Autodesk Inventor part; units mm, degrees
ref_plane "YZ Plane" through (0, 0, 0) normal (1, 0, 0) x (0, 1, 0)
ref_plane "XZ Plane" through (0, 0, 0) normal (0, 1, 0) x (-1, 0, 0)
ref_plane "XY Plane" through (0, 0, 0) normal (0, 0, 1) x (1, 0, 0)
sketch "Sketch1" plane through (0, 0, 0) normal (0, 1, 0) x (-1, 0, 0)
  line L0 (0, -37.5) -> (0, 0)
  line L1 (0, 0) -> (-74.5, 0)
  line L2 (-74.5, 0) -> (-74.5, -18)
  line L3 (-74.5, -18) -> (-15, -37.5)
  line L4 (-15, -37.5) -> (0, -37.5)
  dimension "d0" = 37.5
  dimension "d1" = 74.5
  dimension "d2" = 18
  dimension "d3" = 15
extrude "Extrusion1" add sketch "Sketch1" along normal blind 6.5
sketch "Sketch2" plane through (0, 0, 0) normal (0, -1, 0) x (1, 0, 0)
  line L0 (0, 0) -> (0, -37.5)
  line L1 (0, -37.5) -> (15, -37.5)
  line L2 (16.3, -23.5) -> (16.3, -28)
  line L3 (0, -28) -> (0, -23.5)
  line L4 (5, -21) -> (12.3, -21)
  line L5 (12.3, -30.5) -> (5, -30.5)
  line L6 (0, -23.5) -> (5, -23.5)
  line L7 (12.3, -23.5) -> (16.3, -23.5)
  line L8 (16.3, -28) -> (12.3, -28)
  line L9 (5, -28) -> (0, -28)
  line L10 (5, -30.5) -> (5, -28)
  line L11 (5, -23.5) -> (5, -21)
  line L12 (12.3, -21) -> (12.3, -23.5)
  line L13 (12.3, -28) -> (12.3, -30.5)
  point P0 (16.3, -25.75)
  dimension "d6" = 4.5
  dimension "d7" = 2.5
  dimension "d8" = 5
  dimension "d9" = 7.3
  dimension "d10" = 4
  dimension "d12" = 14
extrude "Extrusion2" cut sketch "Sketch2" against normal through all
sketch "Sketch3" plane through (0, 0, 0) normal (0, -1, 0) x (1, 0, 0)
  line L0 (74.5, -18) -> (74.5, 0)
  line L1 (74.5, 0) -> (0, 0)
  line L2 (66.5, 0) -> (58.5, 0)
  line L3 (58.5, 0) -> (58.5, 4.5)
  line L4 (60.5, 6.5) -> (64.5, 6.5)
  line L5 (66.5, 4.5) -> (66.5, 0)
  arc A0 (60.5, 6.5) -> (58.5, 4.5) centre (60.5, 4.5) ccw
  arc A1 (66.5, 4.5) -> (64.5, 6.5) centre (64.5, 4.5) ccw
  dimension "d15" = 2
  dimension "d16" = 8
  dimension "d17" = 6.5
  dimension "d18" = 8
extrude "Extrusion3" add sketch "Sketch3" against normal blind 6.5
sketch "Sketch4" plane through (0, 0, 0) normal (0, -1, 0) x (1, 0, 0)
  line L0 (58.5, 4.5) -> (58.5, 0)
  line L1 (58.5, 0) -> (0, 0)
  line L2 (48.75, 0) -> (53.25, 0)
  line L3 (53.25, -16.3) -> (48.75, -16.3)
  line L4 (55.75, -5) -> (55.75, -12.3)
  line L5 (46.25, -12.3) -> (46.25, -5)
  line L6 (46.25, -5) -> (48.75, -5)
  line L7 (53.25, -5) -> (55.75, -5)
  line L8 (55.75, -12.3) -> (53.25, -12.3)
  line L9 (48.75, -12.3) -> (46.25, -12.3)
  line L10 (48.75, -16.3) -> (48.75, -12.3)
  line L11 (48.75, -5) -> (48.75, 0)
  line L12 (53.25, 0) -> (53.25, -5)
  line L13 (53.25, -12.3) -> (53.25, -16.3)
  point P0 (51, -16.3)
  dimension "d21" = 4.5
  dimension "d22" = 2.5
  dimension "d23" = 5
  dimension "d24" = 4
  dimension "d25" = 7.3
  dimension "d26" = 7.5
extrude "Extrusion4" cut sketch "Sketch4" against normal through all
sketch "Sketch5" plane through (0, 0, 0) normal (0, -1, 0) x (1, 0, 0)
  line L0 (15, -37.5) -> (74.5, -18)
  line L1 (74.5, -18) -> (74.5, 0)
  line L2 (74.5, 0) -> (66.5, 0)
  arc A0 (71.9111, -18.8485) -> (57.845, -23.4584) centre (64.5, -20) ccw
  dimension "d29" = 15
  dimension "d30" = 20
  dimension "d31" = 10
extrude "Extrusion5" cut sketch "Sketch5" against normal through all
properties part number "x_carryage_brace_bottom"
CAD build for the part. Positions are in the model's coordinates, mm. A direction names the side the tool comes from. Give positions to 0.01 mm unless a question says otherwise; leave off trailing zeros. Loops run counter-clockwise (first coordinate to the right, second up) from the corner with the lowest first, then second, coordinate; pieces in that order, holes last. Notation, with made-up numbers: M 14,20 L 64,20 A17 ccw 64,49 Z; hole C -3,84.5 d8. An arc over 180 degrees is marked long. One line per question, with ' | ' between items. Start each with the question number.
1. Two-plate mould, pull along X, no slides. Class faces 1 (the face through (29, 6.5, -15)), 2 (the face through (48.75, 3, -3)), 3 (the face through (5, 3, -29)), 4 (the face through (0, 3, -12)): pulls with the +X half, pulls with the -X half, needs draft (parallel to the pull), parting line crosses it, or undercut.
2. 3-axis set-ups, long thin cutter, end or side, ignore diameter. For faces 5 (the face through (5, 3, -22)), 6 (the face through (2, 3, -23.5)), 7 (the face through (56, 3, 0)): which of +Z, -Z, +X, -X, +Y, -Y reach the whole face in a straight line?
3. Saw through at C-C on z = -13.5. Give the cut face in (x, y), plus the area to 3 significant figures.
4. Saw through at D-D on x = 38. Give the cut face in (y, z).
5. Probe L1, parallel to Z at x = 4, y = 1.25; L2, parallel to Z at x = 8.5, y = 4.75; L3, parallel to X at y = 2.5, z = -11. List the from-to ranges inside material, lowest first. Write a range as from..to.
6. Flat gauge pins, fed straight in: pin 1 (3 mm diameter, centred on x = 13.5, y = 4.5, fed in from +Z); pin 2 (2 mm diameter, centred on x = 48, y = 4.5, fed in from -Z); pin 3 (3.5 mm diameter, centred on y = 3, z = 2.5, fed in from +X); pin 4 (1 mm diameter, centred on x = 17, z = 1.5, fed in from +Y). Where does each tip first touch, or does it go through?
7. Saw through at B-B on x = 9. Give the cut face in (y, z), plus the area to 3 significant figures.
8. Saw through at A-A on z = -7. Give the cut face in (x, y).
Result sheet:
1) face 1: needs draft | face 2: undercut | face 3: undercut | face 4: pulls with the -X half
2) face 5: +Y, -Y | face 6: -X, +Y, -Y | face 7: +Z, -X, +Y, -Y
3) outline: M 0,0 L 48.75,0 L 48.75,6.5 L 0,6.5 Z; M 53.25,0 L 60.76,0 L 60.76,6.5 L 53.25,6.5 Z; M 68.24,0 L 74.5,0 L 74.5,6.5 L 68.24,6.5 Z | area: 406 mm^2
4) outline: M 0,-29.96 L 6.5,-29.96 L 6.5,0 L 0,0 Z
5) L1: z = -37.5..-28, -23.5..0 | L2: z = -37.5..-30.5, -21..0 | L3: x = 0..46.25, 55.75..74.5
6) pin 1: stops at z = 0 | pin 2: stops at z = -27.01 | pin 3: stops at x = 66.5 | pin 4: passes through
7) outline: M 0,-37.5 L 6.5,-37.5 L 6.5,-30.5 L 0,-30.5 Z; M 0,-21 L 6.5,-21 L 6.5,0 L 0,0 Z | area: 182 mm^2
8) outline: M 0,0 L 46.25,0 L 46.25,6.5 L 0,6.5 Z; M 55.75,0 L 74.5,0 L 74.5,6.5 L 55.75,6.5 Z
